The drawing under review shows one solid part. Ordinate dimensions are in mm from its lowest x, y, z. A direction names the side the tool comes from. Coordinates: 2 decimals unless noted, no trailing zeros. Loops run counter-clockwise (first coordinate to the right, second up) from the corner with the lowest first, then second, coordinate; pieces in that order, holes last. Notation, with made-up numbers: M -24,-11.75 L 20,-11.75 A30 ccw 20,17.25 Z; hole C -25.5,38.25 d6. An arc over 180 degrees is marked long. Use one line per item in the form item = value.
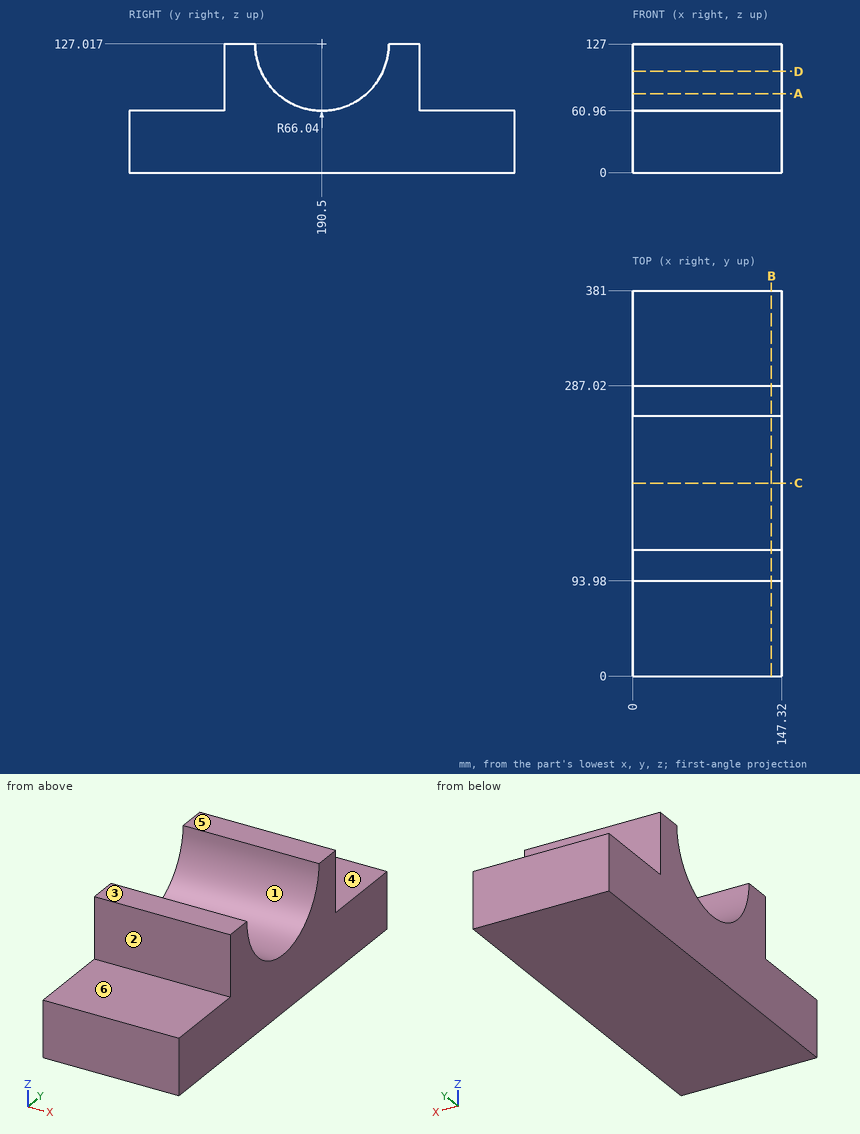
1. Consider section D-D on z = 100. Write out the cut boundary in (x, y).
Computed values:
outline = M 0,93.98 L 147.32,93.98 L 147.32,130.24 L 0,130.24 Z; M 0,250.76 L 147.32,250.76 L 147.32,287.02 L 0,287.02 Z
2. Wall thickness on line 1 along Z through (x, y) = (47, 360); line 2 along Y through (x, z) = (29, 96); line 3 along Y through (x, z) = (135, 75.5): over which ranges is each line inside the solid? List them lowest first. Write a range as from..to.
Computed values:
line_1 = 0..60.96
line_2 = 93.98..132.2, 248.8..287.02
line_3 = 93.98..149.18, 231.82..287.02
3. Draft analysis for pull direction Y (two halves, no side actions). For the marked faces 1, 2 and 3, state which applies: +Y half, -Y half, draft (parallel to the pull), parting line (faces both ways), or undercut.
Computed values:
face_1 = undercut
face_2 = -Y half
face_3 = draft
4. Tool access review of the marked faces 4, 5 and 6: name each direction out of +Z, -Z, +X, -X, +Y, -Y from which nothing blocks a thin tool from reaching the whole face with its end or side.
Computed values:
face_4 = +Z, +X, -X, +Y
face_5 = +Z, +X, -X, +Y, -Y
face_6 = +Z, +X, -X, -Y
5. For pin 1 Ø1.5 at (x, z) = (54, 82.5) entering from -Y; pin 2 Ø10 at (x, y) = (57.5, 138.5) entering from +Z (1 decimal); pin 3 Ø5 at (x, y) = (103.5, 90) entering from +Z, all flat-tipped, find the tip position at first contact; note any pin that passes through.
Computed values:
pin_1 = 93.98
pin_2 = 93.7
pin_3 = 60.96
6. Consider section C-C on y = 190.5. Write out the cut boundary in (x, z).
Computed values:
outline = M 0,0 L 147.32,0 L 147.32,60.98 L 0,60.98 Z
7. Consider section A-A on z = 78. Write out the cut boundary in (x, y) (1 decimal).
Computed values:
outline = M 0,94 L 147.3,94 L 147.3,146.2 L 0,146.2 Z; M 0,234.8 L 147.3,234.8 L 147.3,287 L 0,287 Z
8. Consider section B-B on x = 137. Write out the cut boundary in (y, z), plus the area to 3 significant figures.
Computed values:
outline = M 0,0 L 381,0 L 381,60.96 L 287.02,60.96 L 287.02,127 L 256.54,127 A66.04 cw 124.46,127 L 93.98,127 L 93.98,60.96 L 0,60.96 Z
area = 29,100 mm2
